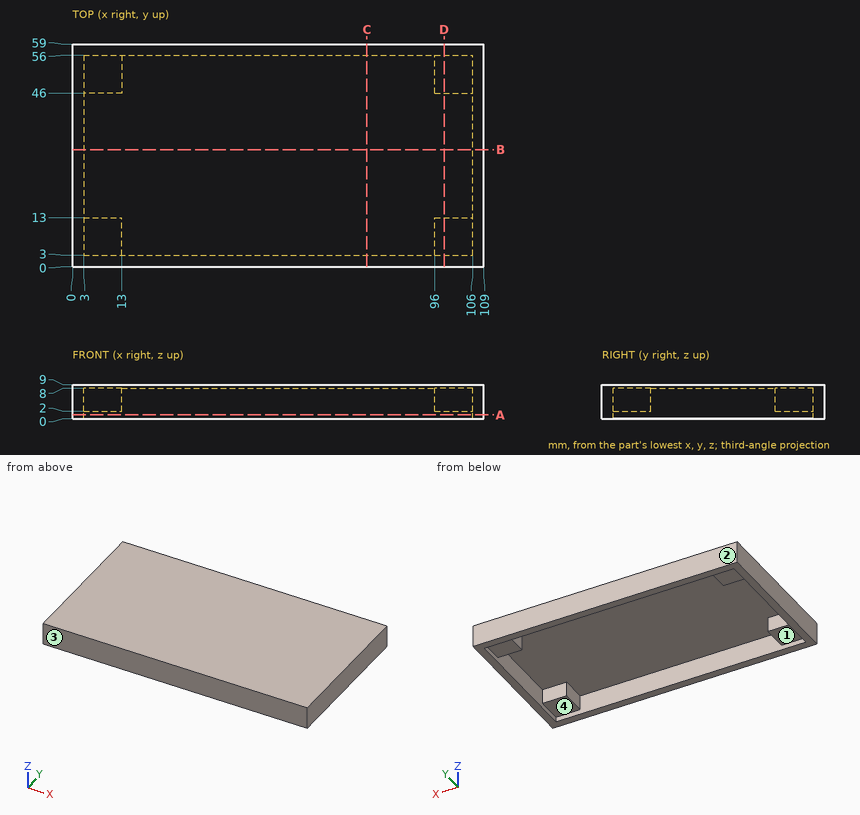
Geometry: see drawing. Coordinates: mm, zero at the bounding-box minimum. A direction names the side the tool comes from. Round coordinates to 2 decimals unless told otherwise and drop trailing zeros. Write each loop counter-clockwise with the first axis right and the second up, starting at its lowest first coordinate (ties: lowest second). Pieces come first, ordered by that corner, then holes. Notation, with made-up numbers: M 36,-39 L 92,-39 A17 ccw 92,-7 Z; hole C -6,41 d8. An arc over 180 degrees is marked long. Answer in a Markdown table with one row per item. Add a question column.
(1) Cut plane D-D, the plane x = 98.5. Return the cut outline in (y, z), then the cut area to 3 significant figures.
(2) Draft query along X for the marked faces 3 and 4. Return one class per face: pulls with the +X half, pulls with the -X half, needs draft (parallel to the pull), parting line crosses it, or undercut.
(3) Cut plane C-C, the plane x = 78. Return the cut outline in (y, z), then the cut area to 3 significant figures.
(4) Contact query for flat-ended pins moving along their axis: pin 1 (5 mm diameter, centred on x = 80, y = 42, fed in from -Z); pin 2 (3 mm diameter, centred on x = 99.5, y = 7.5, fed in from -Z). Output: stop coordinate, or through.
(5) Reachability of the marked faces 1 and 2 from +Z, -Z, +X, -X, +Y, -Y: full face, straight path, thin tool, end or side. Return the list, or none.
(6) Cut plane A-A, the plane z = 1. Return the cut outline in (x, y), then the cut area to 3 significant figures.
(7) Cut plane B-B, the plane y = 31. Return the cut outline in (x, z), then the cut area to 3 significant figures.
(8) Ray query, L1, parallel to X at y = 9.5, z = 6.75; L2, parallel to Y at x = 7.5, z = 1.75; L3, parallel to X at y = 33.5, z = 1. Return the intervals inside material, ascending.
Established:
| question | item | result |
|---|---|---|
| 1 | outline | M 0,0 L 3,0 L 3,2 L 13,2 L 13,8 L 46,8 L 46,2 L 56,2 L 56,0 L 59,0 L 59,9 L 0,9 Z |
| 1 | area | 227 mm² |
| 2 | face 3 | needs draft |
| 2 | face 4 | undercut |
| 3 | outline | M 0,0 L 3,0 L 3,8 L 56,8 L 56,0 L 59,0 L 59,9 L 0,9 Z |
| 3 | area | 107 mm² |
| 4 | pin 1 | z = 8 |
| 4 | pin 2 | z = 2 |
| 5 | face 1 | -Z |
| 5 | face 2 | +Z, -Z, +X, -X, +Y |
| 6 | outline | M 0,0 L 109,0 L 109,59 L 0,59 Z; hole M 3,3 L 106,3 L 106,56 L 3,56 Z |
| 6 | area | 972 mm² |
| 7 | outline | M 0,0 L 3,0 L 3,8 L 106,8 L 106,0 L 109,0 L 109,9 L 0,9 Z |
| 7 | area | 157 mm² |
| 8 | L1 | 0 to 13, 96 to 109 |
| 8 | L2 | 0 to 3, 56 to 59 |
| 8 | L3 | 0 to 3, 106 to 109 |
